```python
from build123d import *

# Parameters (mm, degrees)
F2_DEPTH = 31.75
F0_W     = 50.8
F0_H     = 12.7
F0_R     = 1.651
F3_DEPTH = 12.7
F4_R     = 12.7
F5_R     = 12.69999


# Not quite as in the source:
# - a fillet or chamfer is up to 0.001 mm smaller than in the source, because OpenCascade refuses the exact size


with BuildPart() as f2:
    # F1 (on face) → F2 (new body)
    with BuildSketch(Plane.XY):
        Polygon((12.7, -6.3331015408), (12.7, 6.3278423622), (7.1869615835, 6.35), (-12.7, 6.35), (-12.7, -6.310286466), align=None)
    extrude(amount=F2_DEPTH)

    # F0 (on Top) → F3 (join)
    with BuildSketch(Plane.XY):
        Rectangle(F0_W, F0_H)
        with Locations((-19.05, 0)):
            Circle(F0_R, mode=Mode.SUBTRACT)
        with Locations((19.05, 0)):
            Circle(F0_R, mode=Mode.SUBTRACT)
    extrude(amount=F3_DEPTH)

    # F4
    f4_edges = [f2.edges().sort_by_distance(p)[0] for p in [
        (-12.7, 0.019857, 31.75),
    ]]
    fillet(f4_edges, radius=F4_R)

    # F5 (radius 12.7 in the source; OpenCascade refuses exactly that, so slightly less here)
    f5_edges = [f2.edges().sort_by_distance(p)[0] for p in [
        (12.7, -0.00263, 31.75),
    ]]
    fillet(f5_edges, radius=F5_R)


solid = f2.part
```
Could you check a few things on this model? Use its own coordinates, in mm. A direction names the side the tool comes from. Round coordinates to 2 decimals unless told otherwise and drop trailing zeros. Loops run counter-clockwise (first coordinate to the right, second up) from the corner with the lowest first, then second, coordinate; pieces in that order, holes last. Notation, with made-up numbers: (3.25, 10) - (42.25, 10) arc R29 cw to (42.25, 43) - close; hole circle Ø11 at (4, 22). An arc over 180 degrees is marked (long way). Answer as CSV lines item,"result".
1. Please list where these lines run through material, in increasing order: line 1 along Y through (x, z) = (-19.05, 9.5); line 2 along Y through (x, z) = (-10.5, 24); line 3 along Y through (x, z) = (1.5, 28). Write a range as [from, to].
Filled in:
line 1,"y = [-6.35, -1.65], [1.65, 6.35]"
line 2,"y = [-6.31, 6.35]"
line 3,"y = [-6.32, 6.35]"
2. For pin 1 Ø3 at (x, y) = (-19.05, 0) entering from -Z; pin 2 Ø1 at (x, y) = (-2, 4.5) entering from +Z; pin 3 Ø1.9 at (y, z) = (3, 14.5) entering from -X; pin 4 Ø3 at (y, z) = (4.5, 18) entering from +X, each with a flat end and sliding along its axis, tell me the tip position at first contact or that it passes through.
Filled in:
pin 1,"passes through"
pin 2,"stops at z = 31.66"
pin 3,"stops at x = -12.7"
pin 4,"stops at x = 12.7"
3. I want a section at B-B on y = 0. Count the separate pieces of the cut face and the enclosed holes in it, then the cut area to 3 significant figures.
Filled in:
separate pieces,"3"
enclosed holes,"0"
area,"976 mm^2"
4. We'd pull the mould along Y, two halves only. Please class faces 4 (the face through (17, 0, 12.7)), 5 (the face through (0, -6.35, 6)), 6 (the face through (-20.7, 0.07, 6.26)): +Y half, -Y half, draft (parallel to the pull), parting line (faces both ways), or undercut.
Filled in:
face 4,"draft"
face 5,"-Y half"
face 6,"undercut"
5. On a 3-axis mill with a long thin cutter (end or side, diameter ignored), from which of +Z, -Z, +X, -X, +Y, -Y can I reach the whole of each face in a straight line? I mean faces 1 (the face through (12.7, 0, 16)), 2 (the face through (-12.7, 0, 16)), 3 (the face through (0, 6.35, 12)). Say none if no direction works.
Filled in:
face 1,"+Z, +X, +Y, -Y"
face 2,"+Z, -X, +Y, -Y"
face 3,"+Z, -Z, +X, -X, +Y"
6. I want a section at A-A on x = 19.05. List the corners of the cut face in (y, z) for me, then the cut area to 3 significant figures.
Filled in:
outline,"(-6.35, 0) - (-1.65, 0) - (-1.65, 12.7) - (-6.35, 12.7) - close; (1.65, 0) - (6.35, 0) - (6.35, 12.7) - (1.65, 12.7) - close"
area,"119 mm^2"
7. I want a section at D-D on x = -18. List the corners of the cut face in (y, z) for me, then the cut area to 3 significant figures.
Filled in:
outline,"(-6.35, 0) - (-1.27, 0) - (-1.27, 12.7) - (-6.35, 12.7) - close; (1.27, 0) - (6.35, 0) - (6.35, 12.7) - (1.27, 12.7) - close"
area,"129 mm^2"
